```python
from build123d import *

# Parameters (mm, degrees)
SKETCH1_R           = 12.7
SKETCH1_R_2         = 3.175
BOSS_EXTRUDE1_DEPTH = 10
SKETCH1_3_R         = 12.7
SKETCH1_3_R_2       = 6.35
BOSS_EXTRUDE2_DEPTH = 2.5
SKETCH2_R           = 12.7
BOSS_EXTRUDE3_DEPTH = 10
SKETCH3_R           = 5
CUT_EXTRUDE3_DEPTH  = 10
CUT_EXTRUDE4_START  = -1.45
SKETCH4_R           = 10
CUT_EXTRUDE4_DEPTH  = 5
CUT_EXTRUDE5_DEPTH  = 2


with BuildPart() as part:
    # Sketch1 → Boss-Extrude1 (new body)
    with BuildSketch(Plane(origin=(0, 0, 0), x_dir=(1, 0, 0), z_dir=(0, 1, 0))):
        with BuildLine():
            Line((-41.199040767, 52.757793765), (38.800959233, 52.757793765))
            ThreePointArc((38.800959233, 52.757793765), (45.872027044, 49.828861577), (48.800959233, 42.757793765))
            Line((48.800959233, 42.757793765), (48.800959233, -37.242206235))
            ThreePointArc((48.800959233, -37.242206235), (45.872027044, -44.313274047), (38.800959233, -47.242206235))
            Line((38.800959233, -47.242206235), (-41.199040767, -47.242206235))
            ThreePointArc((-41.199040767, -47.242206235), (-48.270108579, -44.313274047), (-51.199040767, -37.242206235))
            Line((-51.199040767, -37.242206235), (-51.199040767, 42.757793765))
            ThreePointArc((-51.199040767, 42.757793765), (-48.270108579, 49.828861577), (-41.199040767, 52.757793765))
        make_face()
        with Locations(Location((0, 0, 0), (0, 0, 270))):
            Circle(SKETCH1_R, mode=Mode.SUBTRACT)
        with Locations(Location((-41.199040767, 42.757793765, 0), (0, 0, 270))):
            Circle(SKETCH1_R_2, mode=Mode.SUBTRACT)
        with Locations(Location((38.800959233, 42.757793765, 0), (0, 0, 270))):
            Circle(SKETCH1_R_2, mode=Mode.SUBTRACT)
        with Locations(Location((38.800959233, -37.242206235, 0), (0, 0, 270))):
            Circle(SKETCH1_R_2, mode=Mode.SUBTRACT)
        with Locations(Location((-41.199040767, -37.242206235, 0), (0, 0, 270))):
            Circle(SKETCH1_R_2, mode=Mode.SUBTRACT)
    extrude(amount=BOSS_EXTRUDE1_DEPTH)

    # Sketch1<3> → Boss-Extrude2 (add)
    with BuildSketch(Plane(origin=(0, 0, 0), x_dir=(1, 0, 0), z_dir=(0, 1, 0))):
        with Locations(Location((0, 0, 0), (0, 0, 270))):
            Circle(SKETCH1_3_R)
        with Locations(Location((0, 0, 0), (0, 0, 270))):
            Circle(SKETCH1_3_R_2, mode=Mode.SUBTRACT)
    extrude(amount=BOSS_EXTRUDE2_DEPTH)

    # Sketch2 → Boss-Extrude3 (add, through all)
    with BuildSketch(Plane(origin=(0, 10, 0), x_dir=(1, 0, 0), z_dir=(0, 1, 0))):
        Circle(SKETCH2_R)
    extrude(amount=-BOSS_EXTRUDE3_DEPTH)

    # Sketch3 → Cut-Extrude3 (cut)
    with BuildSketch(Plane(origin=(0, 10, 0), x_dir=(1, 0, 0), z_dir=(0, 1, 0))):
        with Locations(Location((-1.199040767, 2.757793765, 0), (0, 0, 270))):
            Circle(SKETCH3_R)
    extrude(amount=-CUT_EXTRUDE3_DEPTH, mode=Mode.SUBTRACT)

    # Sketch4 → Cut-Extrude4 (cut)
    with BuildSketch(Plane(origin=(0, 10, 0), x_dir=(1, 0, 0), z_dir=(0, 1, 0)).offset(CUT_EXTRUDE4_START)):
        with Locations(Location((-1.199040767, 2.757793765, 0), (0, 0, 270))):
            Circle(SKETCH4_R)
    extrude(amount=-CUT_EXTRUDE4_DEPTH, mode=Mode.SUBTRACT)

    # Sketch6 → Cut-Extrude5 (cut)
    with BuildSketch(Plane.XZ):
        with BuildLine():
            Line((48.800959233, -42.757793765), (48.800959233, 37.242206235))
            ThreePointArc((48.800959233, 37.242206235), (45.872027044, 44.313274047), (38.800959233, 47.242206235))
            Line((38.800959233, 47.242206235), (-41.199040767, 47.242206235))
            ThreePointArc((-41.199040767, 47.242206235), (-48.270108579, 44.313274047), (-51.199040767, 37.242206235))
            Line((-51.199040767, 37.242206235), (-51.199040767, -42.757793765))
            ThreePointArc((-51.199040767, -42.757793765), (-48.270108579, -49.828861577), (-41.199040767, -52.757793765))
            Line((-41.199040767, -52.757793765), (38.800959233, -52.757793765))
            ThreePointArc((38.800959233, -52.757793765), (45.872027044, -49.828861577), (48.800959233, -42.757793765))
        make_face()
    extrude(amount=-CUT_EXTRUDE5_DEPTH, mode=Mode.SUBTRACT)


solid = part.part
```
Could you check a few things on this model? Use its own coordinates, in mm. A direction names the side the tool comes from. Coordinates: 2 decimals unless noted, no trailing zeros. Write each loop counter-clockwise with the first axis right and the second up, starting at its lowest first coordinate (ties: lowest second). Pieces come first, ordered by that corner, then holes. Notation, with made-up numbers: (0.5, -1.5) -> (31.5, -1.5) arc R22 ccw to (31.5, 26.5) -> close; hole circle Ø5 at (44, 35). An arc over 180 degrees is marked (long way). One line per question, with ' | ' between items. Start each with the question number.
1. For faces 1 (the face through (3.4, 8.55, -5.1)), 2 (the face through (-1, 6, 47.242)), which set-ups out of +Z, -Z, +X, -X, +Y, -Y let a thin tool reach every point of the face, with its end or its side?
2. If we section it at B-B (z = -41.5): Please give me the cut outline in (x, y), and give its area (3 significant figures).
3. Thinking about a two-plate mould opening in Y: for faces 3 (the face through (1.8, 6.09, 6.78)), 4 (the face through (45.8, 5.9, -49.9)), 5 (the face through (-2, 2, 9)), which applies, pulls with the +Y half, pulls with the -Y half, needs draft (parallel to the pull), parting line crosses it, or undercut?
4. If we section it at A-A (x = -3.5): Please give me the cut outline in (y, z).
5. Please list where these lines run through material, in increasing order: line 1 along X through (y, z) = (5.75, 36.5); line 2 along Z through (x, y) = (40, 7.5); line 3 along X through (y, z) = (8.5, 4.5).
6. If we section it at D-D (z = -2.5): Please give me the cut outline in (x, y), and give its area (3 significant figures).
7. If we section it at C-C (y = 5.5): Please give me the cut outline in (x, z) (3 decimals), and give its area (3 significant figures).
8. Will this pin go through, and if not, where does the flat tip stop? P1, Ø5, axis at x = -41.2, z = 37.24, coming from the -Y side.
Return value:
1) face 1: none | face 2: +Z, +X, -X, +Y, -Y
2) outline: (-51.2, 2) -> (-44.11, 2) -> (-44.11, 10) -> (-51.2, 10) -> close; (-38.28, 2) -> (35.89, 2) -> (35.89, 10) -> (-38.28, 10) -> close; (41.72, 2) -> (48.8, 2) -> (48.8, 10) -> (41.72, 10) -> close | area: 707 mm²
3) face 3: undercut | face 4: needs draft | face 5: pulls with the -Y half
4) outline: (2, -52.76) -> (10, -52.76) -> (10, -7.2) -> (8.55, -7.2) -> (8.55, -12.49) -> (3.55, -12.49) -> (3.55, -7.2) -> (2, -7.2) -> close; (2, 1.68) -> (3.55, 1.68) -> (3.55, 6.97) -> (8.55, 6.97) -> (8.55, 1.68) -> (10, 1.68) -> (10, 47.24) -> (2, 47.24) -> close
5) line 1: x = -51.2 to -44.29, -38.11 to 35.71, 41.89 to 48.8 | line 2: z = -52.69 to -45.7, -39.82 to 34.3, 40.18 to 47.17 | line 3: x = -51.2 to -8.08, 5.68 to 48.8
6) outline: (-51.2, 2) -> (-6.19, 2) -> (-6.19, 3.55) -> (-11.2, 3.55) -> (-11.2, 8.55) -> (-6.19, 8.55) -> (-6.19, 10) -> (-51.2, 10) -> close; (3.79, 2) -> (48.8, 2) -> (48.8, 10) -> (3.79, 10) -> (3.79, 8.55) -> (8.8, 8.55) -> (8.8, 3.55) -> (3.79, 3.55) -> close | area: 670 mm²
7) outline: (-51.199, -42.758) arc R10 ccw to (-41.199, -52.758) -> (38.801, -52.758) arc R10 ccw to (48.801, -42.758) -> (48.801, 37.242) arc R10 ccw to (38.801, 47.242) -> (-41.199, 47.242) arc R10 ccw to (-51.199, 37.242) -> close; hole circle Ø6.35 at (-41.199, -42.758); hole circle Ø6.35 at (-41.199, 37.242); hole circle Ø20 at (-1.199, -2.758); hole circle Ø6.35 at (38.801, -42.758); hole circle Ø6.35 at (38.801, 37.242) | area: 9,470 mm²
8) P1: passes through
